Here's how the part is built. I have some questions about the finished solid (model axes, mm). A direction names the side the tool comes from. Round coordinates to 2 decimals unless told otherwise and drop trailing zeros. Order: outer loops, then holes, each group sorted by start corner. A loop starts at its lowest first (then second) coordinate and runs counter-clockwise, first axis right, second up. Notation, with made-up numbers: (48, 24) - (85, 24) arc R4 cw to (85, 31) - close; hole circle Ø7 at (-18.5, 54.5). An arc over 180 degrees is marked (long way). Answer as a JSON object with one key per item and string values.
```python
from build123d import *

# Parameters (mm, degrees)
F1_DEPTH    = 7.62
F3_DEPTH    = 3.81
F5_DEPTH    = 3.81
F7_D        = 4.7625
F7_DEPTH    = 12.7
F7_TIP      = 1.4307993491
F8_T1_DEPTH = 46.8124487366


# Not quite as in the source:
# - a fillet or chamfer that OpenCascade refuses, or shapes differently, is made with other operations: its cross-section is extruded or revolved along the edge and cut away or added


with BuildPart() as f1:
    # F0 (on Top) → F1 (new body)
    with BuildSketch(Plane.XY):
        with BuildLine():
            Line((6.985, 27.4185502146), (0, 27.4185502146))
            Line((0, 27.4185502146), (0, -23.3814497854))
            ThreePointArc((0, -23.3814497854), (2.0458591334, -18.4423089188), (6.985, -16.3964497854))
            Line((6.985, -16.3964497854), (6.985, 27.4185502146))
        make_face()
        with BuildLine():
            ThreePointArc((6.985, -16.3964497854), (2.0458591334, -18.4423089188), (0, -23.3814497854))
            Line((0, -23.3814497854), (6.985, -23.3814497854))
            Line((6.985, -23.3814497854), (6.985, -16.3964497854))
        make_face()
        with BuildLine():
            Line((6.985, -23.3814497854), (0, -23.3814497854))
            ThreePointArc((0, -23.3814497854), (6.985, -30.3664497854), (13.97, -23.3814497854))
            ThreePointArc((13.97, -23.3814497854), (11.9241408666, -18.4423089188), (6.985, -16.3964497854))
            Line((6.985, -16.3964497854), (6.985, -23.3814497854))
        make_face()
    extrude(amount=F1_DEPTH)

    # F2 (on face) → F3 (cut)
    with BuildSketch(Plane.XY.offset(7.62)):
        with BuildLine():
            ThreePointArc((0, -23.3814497854), (6.985, -30.3664497854), (13.97, -23.3814497854))
            ThreePointArc((13.97, -23.3814497854), (11.9241408666, -18.4423089188), (6.985, -16.3964497854))
            ThreePointArc((6.985, -16.3964497854), (2.0458591334, -18.4423089188), (0, -23.3814497854))
        make_face()
    extrude(amount=-F3_DEPTH, mode=Mode.SUBTRACT)

    # F4 (on face) → F5 (join)
    with BuildSketch(Plane(origin=(0, 0, 0), x_dir=(1, 0, 0), z_dir=(0, 0, -1))):
        with BuildLine():
            Line((0, 37.0080322027), (0, 23.3814497854))
            ThreePointArc((0, 23.3814497854), (1.8603767117, 28.1278653964), (6.4505257418, 30.345971468))
            Line((6.4505257418, 30.345971468), (0, 37.0080322027))
        make_face()
    extrude(amount=-F5_DEPTH)

    # F7
    with Locations(Plane.XY.offset(3.81)):
        with Locations((6.985, -23.3814497854)):
            Hole(F7_D / 2, depth=F7_DEPTH)
            with Locations((0, 0, -(F7_DEPTH + F7_TIP / 2))):  # 118° drill point
                Cone(0, F7_D / 2, F7_TIP, mode=Mode.SUBTRACT)

    # F8: chamfer of 7.62 on 1 edges, made by hand

    # F8_s2 → F8_t1 (cut)
    with BuildSketch(Plane.XY.offset(-19.5962243683)):
        Polygon((-0.635, 27.4185502146), (6.985, 19.7985502146), (6.985, 27.4185502146), align=None)
    extrude(amount=F8_T1_DEPTH, mode=Mode.SUBTRACT)


solid = f1.part
```
1. Imagine slicing it at A-A (x = 8). List the corners of the cut face in (y, z) for me.
Responses:
{"outline": "(-30.29, 0) - (-25.54, 0) - (-25.54, 3.81) - (-30.29, 3.81) - close; (-21.23, 0) - (-16.47, 0) - (-16.47, 3.81) - (-21.23, 3.81) - close"}
2. If I drill on L1, parallel to Y at x = 8.5, z = 1; L2, parallel to X at y = -13.5, z = 3.25 (3 decimals); L3, parallel to Y at x = 6.5, z = 3.75, over which ranges is the centre line in solid material (lowest first)? Write a range as [from, to].
Responses:
{"L1": "[-30.2, -25.22], [-21.54, -16.56]", "L2": "[0, 6.985]", "L3": "[-30.35, -25.71], [-21.05, 20.28]"}
3. Imagine slicing it at C-C (z = 5). List the corners of the cut face in (x, y) for me (3 decimals), plus the area to 3 significant figures.
Responses:
{"outline": "(0, -23.381) arc R6.985 cw to (6.985, -16.396) - (6.985, 19.799) - (0, 26.784) - close", "area": "288 mm2"}
4. For P1, Ø4, axis at x = 4.5, y = -26, coming from the +Z side; P2, Ø1.5, axis at y = -6, z = 1.5, coming from the +X side (3 decimals); P3, Ø3, axis at x = 3.5, z = 2, coming from the +Y side, each with a flat end and sliding along its axis, tell me the tip position at first contact or that it passes through.
Responses:
{"P1": "z = 3.81", "P2": "x = 6.985", "P3": "y = 24.78"}
5. Imagine slicing it at D-D (y = 11.5). List the corners of the cut face in (x, z) for me (3 decimals), plus the area to 3 significant figures.
Responses:
{"outline": "(0, 0) - (6.985, 0) - (6.985, 7.62) - (0, 7.62) - close", "area": "53.2 mm2"}
6. For faces 4 (the face through (2.1, -18.39, 5.74)), 5 (the face through (6.985, 1, 4)), 6 (the face through (3, 2, 7.62)), which set-ups out of +Z, -Z, +X, -X, +Y, -Y let a thin tool reach every point of the face, with its end or its side?
Responses:
{"face 4": "+Z, +X, -Y", "face 5": "+Z, -Z, +X, +Y", "face 6": "+Z, +X, -X, +Y, -Y"}
7. Thinking about a two-plate mould opening in Y: for faces 1 (the face through (0, -6, 4)), 2 (the face through (3.444, 23.34, 3.757)), 3 (the face through (5.9, -25.5, 1.9)), which applies, pulls with the +Y half, pulls with the -Y half, needs draft (parallel to the pull), parting line crosses it, or undercut?
Responses:
{"face 1": "needs draft", "face 2": "pulls with the +Y half", "face 3": "undercut"}
8. Imagine slicing it at B-B (y = -24.5). List the corners of the cut face in (x, z) for me, plus the area to 3 significant figures.
Responses:
{"outline": "(0, 0) - (4.88, 0) - (4.88, 3.81) - (0, 3.81) - close; (9.09, 0) - (13.88, 0) - (13.88, 3.81) - (9.09, 3.81) - close", "area": "36.9 mm2"}
